Can you work these out from the model? Positions are in its coordinate system, mm. A direction names the side the tool comes from. Coordinates: 2 decimals unless noted, no trailing zeros. Write each loop counter-clockwise with the first axis right and the second up, starting at its lowest first coordinate (ties: lowest second). Pieces come first, ordered by that corner, then holes. Notation, with made-up numbers: M 25.25,58 L 71.25,58 A3 ccw 71.25,63 Z; hole C 31,85.25 d2. An arc over 180 degrees is marked long. Use one line per item in the form item = value. Start each with the question number.
```python
from build123d import *

# Parameters (mm, degrees)
BOX022_W     = 2
BOX022_H     = 10
BOX022_DEPTH = 9
BOX024_W     = 6
BOX024_H     = 14
BOX024_DEPTH = 1


with BuildPart() as obj1_c:
    # Box022 → Box022 (new body)
    with BuildSketch(Plane(origin=(8.6, 93.3, 10.1), x_dir=(1, 0, 0), z_dir=(0, 0, 1))):
        with Locations((1, 5)):
            Rectangle(BOX022_W, BOX022_H)
    extrude(amount=BOX022_DEPTH)


with BuildPart() as obj1:
    # Box024 → Box024 (new body)
    with BuildSketch(Plane(origin=(6.6, 91.3, 10.1), x_dir=(1, 0, 0), z_dir=(0, 0, 1))):
        with Locations((3, 7)):
            Rectangle(BOX024_W, BOX024_H)
    extrude(amount=BOX024_DEPTH)

    # Fusion037: union obj1_c
    add(obj1_c.part)


solid = obj1.part
```
1) Suppose I cut it at A-A on y = 97.5. Please give me the cut outline in (x, z).
2) Will these pins go through, and if not, where does the flat tip stop? pin 1 Ø1.5 at (x, y) = (7.5, 101.5) entering from +Z; pin 2 Ø1 at (x, z) = (9, 13.5) entering from +Y; pin 3 Ø2 at (x, z) = (8.5, 15.5) entering from -Y.
3) Please list where these lines run through material, in increasing order: line 1 (X direction, y = 100.25, z = 14); line 2 (Y direction, x = 8.65, z = 17.25); line 3 (Z direction, x = 9.25, y = 104.5).
4) Which directions (+Z, -Z, +X, -X, +Y, -Y) give clear straight access to the entire face, cutting with the end or side of a thin tool? Please do faces 1 (the face through (8.6, 98, 15)), 2 (the face through (6.6, 98.2, 10.6)), 3 (the face through (10.6, 98, 15)), 4 (the face through (10, 103.3, 15)), 5 (the face through (10, 93.3, 15)).
5) Suppose I cut it at B-B on x = 9.4. Please give me the cut outline in (y, z), and give its area (3 significant figures).
6) Suppose I cut it at C-C on z = 17.25. Please give me the cut outline in (x, y).
7) Suppose I cut it at D-D on x = 10.8. Please give me the cut outline in (y, z), and give its area (3 significant figures).
Computed values:
q1.outline = M 6.6,10.1 L 12.6,10.1 L 12.6,11.1 L 10.6,11.1 L 10.6,19.1 L 8.6,19.1 L 8.6,11.1 L 6.6,11.1 Z
q2.pin_1 = 11.1
q2.pin_2 = 103.3
q2.pin_3 = 93.3
q3.line_1 = 8.6 to 10.6
q3.line_2 = 93.3 to 103.3
q3.line_3 = 10.1 to 11.1
q4.face_1 = +Z, -X, +Y, -Y
q4.face_2 = +Z, -Z, -X, +Y, -Y
q4.face_3 = +Z, +X, +Y, -Y
q4.face_4 = +Z, +X, -X, +Y
q4.face_5 = +Z, +X, -X, -Y
q5.outline = M 91.3,10.1 L 105.3,10.1 L 105.3,11.1 L 103.3,11.1 L 103.3,19.1 L 93.3,19.1 L 93.3,11.1 L 91.3,11.1 Z
q5.area = 94.0 mm²
q6.outline = M 8.6,93.3 L 10.6,93.3 L 10.6,103.3 L 8.6,103.3 Z
q7.outline = M 91.3,10.1 L 105.3,10.1 L 105.3,11.1 L 91.3,11.1 Z
q7.area = 14.0 mm²
